Here's how the part is built. I have some questions about the finished solid (model axes, mm). Give positions to 0.01 mm unless a question says otherwise; leave off trailing zeros. Loops run counter-clockwise (first coordinate to the right, second up) from the corner with the lowest first, then second, coordinate; pieces in that order, holes last. Notation, with made-up numbers: (85, 58) - (109, 58) arc R28 cw to (109, 90) - close; hole circle Ø10 at (39.5, -23). An arc over 180 degrees is marked (long way). One line per item, written item: value. Start each with the question number.
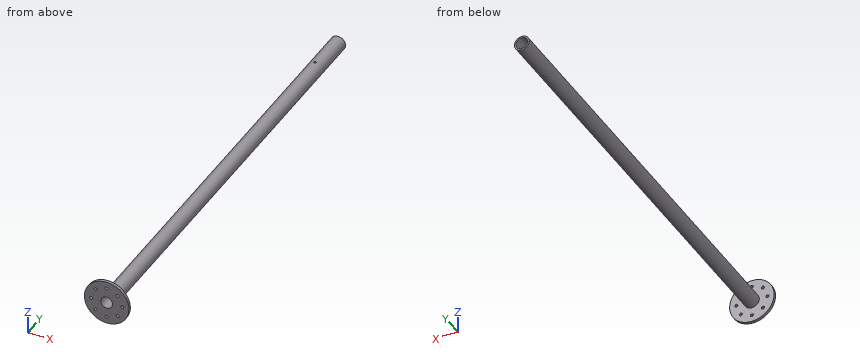
```python
from build123d import *

# Parameters (mm, degrees)
SKETCH1_R                      = 16.7
SKETCH1_R_2                    = 13.32
BOSS_EXTRUDE1_DEPTH            = 1000
SKETCH13_R                     = 50
SKETCH13_R_2                   = 16.7
BOSS_EXTRUDE2_DEPTH            = 6.35
F_1_4_CLEARANCE_HOLE1_D        = 6.7564
F_1_4_CLEARANCE_HOLE1_DEPTH    = 50
F_8_0_199_DIAMETER_HOLE6_D     = 5.0546
F_8_0_199_DIAMETER_HOLE6_DEPTH = 50


with BuildPart() as part:
    # Sketch1 → Boss-Extrude1 (new body)
    with BuildSketch(Plane(origin=(0, 0, 0), x_dir=(1, 0, 0), z_dir=(0, 1, 0))):
        Circle(SKETCH1_R)
        Circle(SKETCH1_R_2, mode=Mode.SUBTRACT)
    extrude(amount=BOSS_EXTRUDE1_DEPTH)

    # Sketch13 → Boss-Extrude2 (add)
    with BuildSketch(Plane(origin=(0, 0, 0), x_dir=(-1, 0, 0), z_dir=(0, -1, 0))):
        Circle(SKETCH13_R)
        Circle(SKETCH13_R_2, mode=Mode.SUBTRACT)
    extrude(amount=-BOSS_EXTRUDE2_DEPTH)

    # 1/4 Clearance Hole1
    with Locations(Plane(origin=(0, 0, 0), x_dir=(-1, 0, 0), z_dir=(0, -1, 0))):
        with Locations((-35, 0), (0, 35), (35, 0), (0, -35), (24.748737342, 24.748737342), (24.748737342, -24.748737342), (-24.748737342, -24.748737342), (-24.748737342, 24.748737342)):
            Hole(F_1_4_CLEARANCE_HOLE1_D / 2, depth=F_1_4_CLEARANCE_HOLE1_DEPTH)

    # #8 (0.199) Diameter Hole6
    with Locations(Plane(origin=(0, 900, -16.7), x_dir=(-1, 0, 0), z_dir=(0, 0, -1))):
        with Locations((0, 0)):
            Hole(F_8_0_199_DIAMETER_HOLE6_D / 2, depth=F_8_0_199_DIAMETER_HOLE6_DEPTH)


solid = part.part
```
(1) Will these pins go through, and if not, where does the flat tip stop? pin 1 (8 mm diameter, centred on x = 13, y = 197, fed in from +Z); pin 2 (4 mm diameter, centred on x = 0, z = -35, fed in from +Y); pin 3 (6.5 mm diameter, centred on x = 0, y = 900, fed in from +Z); pin 4 (8 mm diameter, centred on x = 24.75, z = 24.75, fed in from +Y).
(2) If we section it at A-A on y = 502: List the corners of the cut face in (x, z) for me.
(3) Please list where these lines run through material, in increasing order: probe 1 along Z at (x, y) = (-0.5, 223); probe 2 along Y at (x, z) = (7, 25); probe 3 along Y at (x, z) = (0, -15). Write a range as from..to.
Found:
1. pin 1: z = 14.07
1. pin 2: through
1. pin 3: z = 16.7
1. pin 4: y = 6.35
2. outline: circle Ø33.4 at (0, 0); hole circle Ø26.64 at (0, 0)
3. probe 1: -16.69..-13.31, 13.31..16.69
3. probe 2: 0..6.35
3. probe 3: 0..897.47, 902.53..1000
